Can you work these out from the model? Positions are in its coordinate system, mm. Face numbers are marked on the shaded views. A direction names the side the tool comes from. Give positions to 0.01 mm unless a question says otherwise; leave off trailing zeros. Order: outer loops, then holes, each group sorted by start corner. A loop starts at its lowest first (then second) coordinate and runs counter-clockwise, first axis right, second up. Notation, with made-up numbers: (40.5, -38.5) - (73.5, -38.5) arc R25 cw to (73.5, -4.5) - close; hole circle Ø8 at (-20.5, -8). An arc over 180 degrees is marked (long way). One line per question, with ' | ' between items.
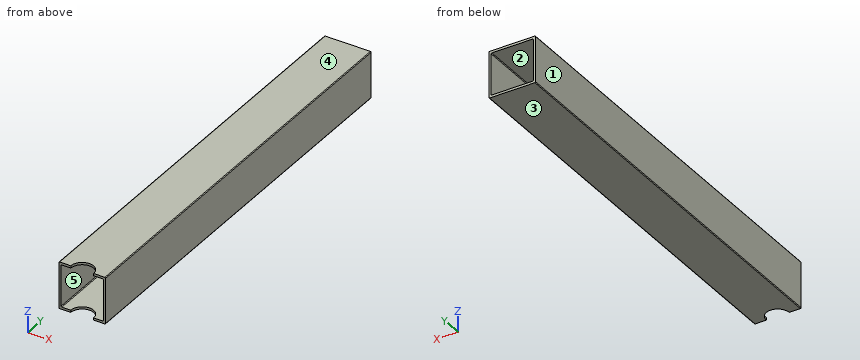
```python
from build123d import *

# Parameters (mm, degrees)
SKETCH1_W           = 25.4
SKETCH1_H           = 25.4
SKETCH1_W_2         = 22.9108
SKETCH1_H_2         = 22.9108
BOSS_EXTRUDE1_DEPTH = 228.6
FILLET1_R           = 0.4064
SKETCH2_R           = 6.19125
CUT_EXTRUDE1_DEPTH  = 232.40501291


with BuildPart() as part:
    # Sketch1 → Boss-Extrude1 (new body)
    with BuildSketch(Plane(origin=(0, 0, 0), x_dir=(1, 0, 0), z_dir=(0, 1, 0))):
        with Locations((12.7, 12.7)):
            Rectangle(SKETCH1_W, SKETCH1_H)
        with Locations((12.7, 12.7)):
            Rectangle(SKETCH1_W_2, SKETCH1_H_2, mode=Mode.SUBTRACT)
    extrude(amount=-BOSS_EXTRUDE1_DEPTH)

    # Fillet1
    fillet1_edges = [part.edges().sort_by_distance(p)[0] for p in [
        (1.2446, -114.3, -1.2446),
        (1.2446, -114.3, -24.1554),
        (24.1554, -114.3, -24.1554),
        (24.1554, -114.3, -1.2446),
        (0, -114.3, -25.4),
        (25.4, -114.3, -25.4),
        (25.4, -114.3, 0),
        (0, -114.3, 0),
    ]]
    fillet(fillet1_edges, radius=FILLET1_R)

    # Sketch2 → Cut-Extrude1 (cut, through all)
    with BuildSketch(Plane(origin=(0, 0, -25.4), x_dir=(-1, 0, 0), z_dir=(0, 0, -1))):
        with Locations((-12.7, -228.6)):
            Circle(SKETCH2_R)
    extrude(amount=-CUT_EXTRUDE1_DEPTH, mode=Mode.SUBTRACT)


solid = part.part
```
(1) Imagine slicing it at B-B (x = 12.7). List the corners of the cut face in (y, z) for me.
Answer below:
outline: (-222.41, -25.4) - (0, -25.4) - (0, -24.16) - (-222.41, -24.16) - close; (-222.41, -1.24) - (0, -1.24) - (0, 0) - (-222.41, 0) - close
(2) If we mould it in two halves opening along X, with no side actions, what happens to the marked faces 1, 2 and 3? For each: released by +X, released by -X, zero draft, split by the parting line, or undercut.
Answer below:
face 1: released by -X | face 2: undercut | face 3: zero draft
(3) Imagine slicing it at A-A (z = -15). List the corners of the cut face in (x, y) for me, and give its area (3 significant figures).
Answer below:
outline: (0, -228.6) - (1.24, -228.6) - (1.24, 0) - (0, 0) - close; (24.16, -228.6) - (25.4, -228.6) - (25.4, 0) - (24.16, 0) - close | area: 569 mm^2
(4) If I drill on line 1 (Z direction, x = 22.25, y = -77.5); line 2 (X direction, y = -112.5, z = -14), over which ranges is the centre line in solid material (lowest first)?
Answer below:
line 1: -25.4 to -24.16, -1.24 to 0 | line 2: 0 to 1.24, 24.16 to 25.4
(5) Imagine slicing it at C-C (y = -132). List the corners of the cut face in (x, z) for me, and give its area (3 significant figures).
Answer below:
outline: (0, -24.99) arc R0.41 ccw to (0.41, -25.4) - (24.99, -25.4) arc R0.41 ccw to (25.4, -24.99) - (25.4, -0.41) arc R0.41 ccw to (24.99, 0) - (0.41, 0) arc R0.41 ccw to (0, -0.41) - close; hole (1.24, -23.75) arc R0.41 ccw to (1.65, -24.16) - (23.75, -24.16) arc R0.41 ccw to (24.16, -23.75) - (24.16, -1.65) arc R0.41 ccw to (23.75, -1.24) - (1.65, -1.24) arc R0.41 ccw to (1.24, -1.65) - close | area: 120 mm^2
(6) On a 3-axis mill with a long thin cutter (end or side, diameter ignored), from which of +Z, -Z, +X, -X, +Y, -Y can I reach the whole of each face in a straight line? I mean the marked faces 4 and 5. Say none if no direction works.
Answer below:
face 4: +Z, +X, -X, +Y, -Y | face 5: +Y, -Y
